Source: CAD feature listing. Evaluate the final solid. Frame: model axes, mm. A direction names the side the tool comes from. Give positions to 0.01 mm unless a question says otherwise; leave off trailing zeros. Write each loop counter-clockwise with the first axis right and the second up, starting at its lowest first coordinate (ties: lowest second). Pieces come first, ordered by that corner, then holes. Notation, with made-up numbers: (58, -9.75) - (107, -9.75) arc R12 ccw to (107, -5.75) - close; hole circle Ø3 at (79.5, -8). An arc over 180 degrees is marked (long way). One line per question, with ' | ' between items. Start each with the question number.
(1) Pin query (flat end, axial travel): pin 1 (1.5 mm diameter, centred on y = 19, z = 3, fed in from -X); pin 2 (17.5 mm diameter, centred on x = -11, y = 24, fed in from +Z); pin 3 (1.5 mm diameter, centred on x = -15, z = -0.5, fed in from +Y). Return the tip coordinate at first contact, or that it passes through.
(2) Access query for faces 1 (the flat face through (-24.54, 16.464, -5.365)), 2 (the cylindrical face through (-5, 10, -5)), 3 (the flat face through (-24.967, 3.493, -5.365)), 4 (the flat face through (-22, 5, 0)), 5 (the flat face through (-10, 23, 0)). Directions: +Z, -Z, +X, -X, +Y, -Y. A direction counts if a zero-diameter tool reaches every point of the face in a straight line with its end or side. Return the directions, or none.
(3) Section B-B, the plane y = 6. Return loops of the section in (x, z), plus the area to 3 significant figures.
(4) Section A-A, the plane z = 1. Return loops of the section in (x, y).
(5) Section C-C, the plane x = -27.5. Return loops of the section in (y, z), plus the area to 3 significant figures.
(6) Ray query, line 1 (Z direction, x = -32, y = 8.5); line 2 (X direction, y = 8.5, z = -2); line 3 (Z direction, x = -36, y = 16). Return the intervals inside material, ascending. Write a range as [from, to].
(7) Section D-D, the plane y = 22. Return loops of the section in (x, z), plus the area to 3 significant figures.
(8) Draft query along Y for faces 6 (the cylindrical face through (-10.54, 12.44, -0.04)), 7 (the flat face through (-5, 35, 0)), 8 (the flat face through (-18, 0, 0)). Return one class per face: +Y half, -Y half, draft (parallel to the pull), parting line (faces both ways), or undercut.
Autodesk Inventor part; units mm, degrees
ref_plane "YZ Plane" through (0, 0, 0) normal (1, 0, 0) x (0, 1, 0)
ref_plane "XZ Plane" through (0, 0, 0) normal (0, 1, 0) x (-1, 0, 0)
ref_plane "XY Plane" through (0, 0, 0) normal (0, 0, 1) x (1, 0, 0)
sketch "Boceto1" plane through (0, 0, 0) normal (0, 0, 1) x (1, 0, 0)
  line L0 (-35, 0) -> (15, 0)
  line L1 (-20, 10) -> (-20, 0)
  arc A0 (-10, 20) -> (-20, 10) centre (-10, 10) ccw
  arc A1 (-10, 25) -> (-25, 10) centre (-10, 10) ccw
  line L2 (-25, 10) -> (-25, 0)
  arc A2 (-10, 35) -> (-35, 10) centre (-10, 10) ccw
  line L3 (-35, 10) -> (-35, 0)
  line L4 (-35, 0) -> (-10, 0)
  circle A3 centre (-10, 10) radius 2.5
  line L5 (-10, 20) -> (0, 20)
  line L6 (0, 20) -> (0, 21.1803)
  line L7 (0, 25) -> (-10, 25)
  line L8 (-10, 35) -> (0, 35)
  line L9 (0, 35) -> (0, 25)
  line L10 (0, 20) -> (0, 0)
  line L11 (0, 0) -> (-10, 0)
  line L12 (0, 25) -> (0, 20)
  line L13 (-10, 25) -> (-10, 20)
  line L14 (-20, 5) -> (-25, 5)
  point P0 (0, 0)
  dimension "d0" = 20
  dimension "d1" = 25
  dimension "d2" = 10
  dimension "d3" = 10
  dimension "d4" = 5
  dimension "d6" = 35
extrude "Extrusión1" add sketch "Boceto1" along normal mid plane 5 contours L3 A2 L8 L9 L7 A1 L2 L0 | L2 L14 L1 L0 | L1 A0 L5 L10 L0 | L7 L12 L6 L5 L13
sketch "Boceto2" plane through (0, 0, 2.5) normal (0, 0, 1) x (1, 0, 0)
  circle A0 centre (-10, 10) radius 2.3
  circle A1 centre (-22.5, 10) radius 2.3
  circle A2 centre (-10, 10) radius 2.5
  point P0 (0, 0)
  dimension "d9" = 4.6
  dimension "d10" = 4.6
extrude "Extrusión2" add sketch "Boceto2" along normal blind 0.4 and the other way blind 5.4 contours A0 | A1
sketch "Boceto3" plane through (-10, 10, 2.9) normal (0, 0, 1) x (1, 0, 0)
  arc A0 (5, 0) -> (0.4927, 4.9757) centre (0, 0) ccw
  line L0 (-30, 0) -> (-30, 7.9951)
  line L1 (0.4927, 4.9757) -> (-30, 7.9951)
  line L2 (-30, 0) -> (-30, -7.9951)
  line L3 (0.4927, -4.9757) -> (-30, -7.9951)
  arc A1 (0.4927, -4.9757) -> (5, 0) centre (0, 0) ccw
  circle A2 centre (0, 0) radius 2.3
  point P0 (10, -10)
  dimension "d15" = 10
extrude "Extrusión3" add sketch "Boceto3" along normal blind 5 contours A1 L3 L2 L0 L1 A0 | A2
sketch "Boceto4" plane through (-22.5, 10, -2.9) normal (0, 0, -1) x (-1, 0, 0)
  circle A0 centre (0, 0) radius 2.3
  circle A1 centre (-12.5, 0) radius 2.3
  line L0 (-12.9927, 4.9757) -> (17.5, 7.9951)
  arc A2 (-12.9927, 4.9757) -> (-12.9927, -4.9757) centre (-12.5, 0) ccw
  line L1 (17.5, -7.9951) -> (-12.9927, -4.9757)
  line L2 (17.5, 7.9951) -> (17.5, -7.9951)
  point P0 (-22.5, -10)
extrude "Extrusión4" add sketch "Boceto4" along normal blind 5 contours A0 | A1 | L0 L2 L1 A2
sketch "Boceto5" plane through (0, 0, -2.5) normal (0, 0, -1) x (-1, 0, 0)
  arc A0 (9.5073, 14.9757) -> (9.5073, 5.0243) centre (10, 10) ccw construction
  circle A1 centre (5, 10) radius 0.4
  circle A2 centre (9.5073, 14.9757) radius 0.4
  line L0 (9.5073, 14.9757) -> (40, 17.9951)
  circle A3 centre (13.4878, 15.3698) radius 0.4
  circle A4 centre (17.4684, 15.764) radius 0.4
  circle A5 centre (21.4489, 16.1581) radius 0.4
  circle A6 centre (25.4294, 16.5523) radius 0.4
  circle A7 centre (29.41, 16.9465) radius 0.4
  circle A8 centre (33.3905, 17.3406) radius 0.4
  line L1 (-2.4318, 10) -> (67.5847, 10) construction
  arc A9 (9.5073, 14.9757) -> (9.5073, 5.0243) centre (10, 10) ccw
  circle A10 centre (9.5073, 5.0243) radius 0.4
  line L2 (9.5073, 5.0243) -> (40, 2.0049)
  circle A11 centre (13.4878, 4.6302) radius 0.4
  circle A12 centre (17.4684, 4.236) radius 0.4
  circle A13 centre (21.4489, 3.8419) radius 0.4
  circle A14 centre (25.4294, 3.4477) radius 0.4
  circle A15 centre (29.41, 3.0535) radius 0.4
  circle A16 centre (33.3905, 2.6594) radius 0.4
  circle A17 centre (10, 10) radius 0.4
  circle A18 centre (14, 10) radius 0.4
  circle A19 centre (18, 10) radius 0.4
  circle A20 centre (22, 10) radius 0.4
  circle A21 centre (26, 10) radius 0.4
  circle A22 centre (30, 10) radius 0.4
  circle A23 centre (34, 10) radius 0.4
  point P0 (0, 0)
  dimension "d45" = 0.8
  dimension "d46" = 0.8
  dimension "d49" = 4
  dimension "d54" = 0.8
  dimension "d57" = 4
extrude "Extrusión5" add sketch "Boceto5" against normal up to surface (5.4 mm away) contours A1 A9 | A16 L2 | L2 A16 | A15 L2 | L2 A15 | A14 L2 | L2 A14 | A13 L2 | L2 A13 | A12 L2 | L2 A12 | A11 L2 | L2 A11 | A10 L2 A9 | A9 L2 A10 | A8 L0 | L0 A8 | A7 L0 | L0 A7 | A6 L0 | L0 A6 | A4 L0 | L0 A4 | A3 L0 | L0 A3 | A2 L0 A9 | A9 L0 A2 | A9 A1 | A18 | A19 | A21 | A22 | A23
mirror "Simetría1" about plane through (0, 0, 0) normal (0, 0, 1) of "Extrusión5"
properties part number "Prueba de soportes mecanismo_3DPrint"
Check sheet entries:
1) pin 1: x = -33.53 | pin 2: z = 2.9 | pin 3: y = 34.64
2) face 1: -Z, +X, +Y | face 2: -Z, +X | face 3: -Z, +X, -Y | face 4: none | face 5: +Z, -Z
3) outline: (-40, -7.9) - (-7, -7.9) - (-7, -2.9) - (-40, -2.9) - close; (-40, 2.9) - (-7, 2.9) - (-7, 7.9) - (-40, 7.9) - close; (-35, -2.5) - (-25, -2.5) - (-25, 2.5) - (-35, 2.5) - close; (-20, -2.5) - (0, -2.5) - (0, 2.5) - (-20, 2.5) - close | area: 480 mm²
4) outline: (-35, 0) - (0, 0) - (0, 35) - (-10, 35) arc R25 ccw to (-35, 10) - close; circle Ø4.6 at (-22.5, 10); circle Ø4.6 at (-10, 10); hole (-25, 5) - (-20, 5) - (-20, 10) arc R10 cw to (-10, 20) - (-10, 25) arc R15 ccw to (-25, 10) - close; hole circle Ø5 at (-10, 10)
5) outline: (0, -2.5) - (27.85, -2.5) - (27.85, 2.5) - (0, 2.5) - close; (3.24, -7.9) - (16.76, -7.9) - (16.76, -2.9) - (3.24, -2.9) - close; (3.24, 2.9) - (16.76, 2.9) - (16.76, 7.9) - (3.24, 7.9) - close | area: 274 mm²
6) line 1: [-7.9, -2.9], [-2.5, 2.5], [2.9, 7.9] | line 2: [-35, -25], [-24.24, -20.76], [-20, -12], [-11.74, -8.26], [-8, 0] | line 3: [-7.9, -2.9], [2.9, 7.9]
7) outline: (-31.93, -2.5) - (-19, -2.5) - (-19, 2.5) - (-31.93, 2.5) - close; (-10, -2.5) - (0, -2.5) - (0, 2.5) - (-10, 2.5) - close | area: 115 mm²
8) face 6: undercut | face 7: +Y half | face 8: -Y half
